from build123d import *

# Parameters (mm, degrees)
F0_W     = 100
F0_H     = 100
F1_DEPTH = 100
F4_R     = 25
F5_DEPTH = 50
F8_D     = 50


# Not quite as in the source:
# - the program builds the solid bodies; features that only make, move or delete a surface that nothing else refers to are left out


with BuildPart() as f1:
    # F0 (on Front) → F1 (new body)
    with BuildSketch(Plane.XZ):
        with Locations((50, 50)):
            Rectangle(F0_W, F0_H)
    extrude(amount=F1_DEPTH)

    # F4 (on face) → F5 (join)
    with BuildSketch(Plane.XY.offset(100)):
        with Locations((49.1654276848, -53.809389472)):
            Circle(F4_R)
    extrude(amount=F5_DEPTH)

    # F8 (through all)
    with Locations(Plane(origin=(0, 0, 0), x_dir=(-1, 0, 0), z_dir=(0, 1, 0))):
        with Locations((-42.2243028879, 47.1359044313)):
            Hole(F8_D / 2)


solid = f1.part
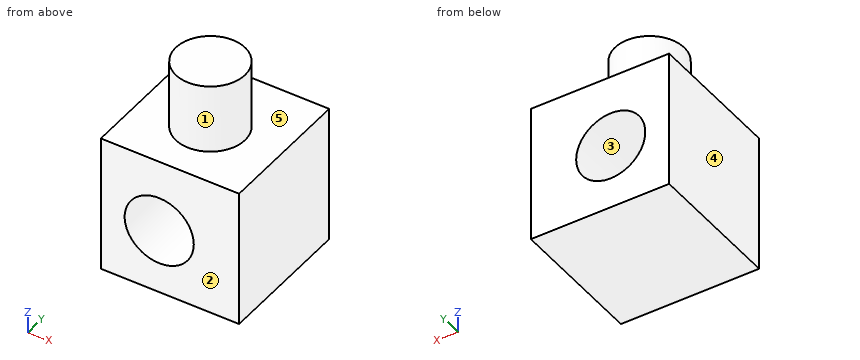
Work out the finished part from the listing and answer in its coordinate system (mm). Face numbers are marked on the shaded views. A direction names the side the tool comes from. Give positions to 0.01 mm unless a question says otherwise; leave off trailing zeros. Write each loop counter-clockwise with the first axis right and the second up, starting at its lowest first coordinate (ties: lowest second). Pieces come first, ordered by that corner, then holes. Notation, with made-up numbers: M 52.25,52 L 103.25,52 A36 cw 103.25,91 Z; hole C -39,-14.75 d3. An arc over 180 degrees is marked long. Answer as CSV lines item,"result".
Q1. Find the intervals of material crossed by probe 1 along X at (y, z) = (-86.5, 46); probe 2 along Z at (x, y) = (95.5, -21.5); probe 3 along Z at (x, y) = (42, -48), in increasing order. Write a range as [from, to].
A:
probe 1,"x = [0, 17.25], [67.2, 100]"
probe 2,"z = [0, 100]"
probe 3,"z = [0, 22.14], [72.13, 150]"
Q2. The mould has two halves that part along X. Classify the marked faces 3, 4 and 5: +X half, -X half, draft (parallel to the pull), parting line (faces both ways), or undercut.
A:
face 3,"undercut"
face 4,"-X half"
face 5,"draft"
Q3. Given P1, Ø1, axis at x = 32.5, z = 26.5, coming from the -Y side, flat-ended and moving along its own axis, determine where the tip first touches the part or whether it passes through.
A:
P1,"passes through"
Q4. A cutting plane is placed at D-D on y = -31. Write down the section's boundary in (x, z), plus the area to 3 significant figures.
A:
outline,"M 0,0 L 100,0 L 100,100 L 59.4,100 L 59.4,150 L 38.93,150 L 38.93,100 L 0,100 Z; hole C 42.22,47.14 d50"
area,"9,060 mm²"
Q5. A cutting plane is placed at A-A on y = -51. Write down the section's boundary in (x, z), plus the area to 3 significant figures.
A:
outline,"M 0,0 L 100,0 L 100,100 L 74.01,100 L 74.01,150 L 24.32,150 L 24.32,100 L 0,100 Z; hole C 42.22,47.14 d50"
area,"10,500 mm²"
Q6. A cutting plane is placed at B-B on x = 45. Write down the section's boundary in (y, z).
A:
outline,"M -100,0 L 0,0 L 0,22.29 L -100,22.29 Z; M -100,71.98 L 0,71.98 L 0,100 L -29.16,100 L -29.16,150 L -78.46,150 L -78.46,100 L -100,100 Z"
Q7. A tool of negligible diameter and unlimited length cuts with its end or side. For the marked faces 1 and 2, from which of +Z, -Z, +X, -X, +Y, -Y can it reach the whole face along a straight path? Write none if from no direction.
A:
face 1,"+Z"
face 2,"+Z, -Z, +X, -X, -Y"
Q8. A cutting plane is placed at C-C on x = 88. Write down the section's boundary in (y, z).
A:
outline,"M -100,0 L 0,0 L 0,100 L -100,100 Z"
